Can you work these out from the model? Positions are in its coordinate system, mm. Give positions to 0.01 mm unless a question says otherwise; leave off trailing zeros. Order: outer loops, then holes, each group sorted by start corner. A loop starts at its lowest first (then second) coordinate and runs counter-clockwise, first axis right, second up. Notation, with made-up numbers: (-8.75, -37.75) - (22.25, -37.75) arc R27 cw to (22.25, -15.75) - close; hole circle Ø3 at (57, 33.25). An arc over 180 degrees is marked (long way). Answer as a JSON object with one key per item and string values.
```python
from build123d import *


with BuildPart() as f1:
    # F0 (on Top) → F1 (revolve)
    with BuildSketch(Plane.XY):
        with BuildLine():
            Line((-2.874578, 26.07), (0, 26.07))
            Line((0, 26.07), (0, 32))
            Line((0, 32), (0, 38.59))
            ThreePointArc((0, 38.59), (-6.422881, 33.474686), (-2.874578, 26.07))
        make_face()
        with BuildLine():
            Line((-8, 0), (0, 0))
            Line((0, 0), (0, 26.07))
            Line((0, 26.07), (-2.874578, 26.07))
            ThreePointArc((-2.874578, 26.07), (-3.059702, 17.543878), (-6.78, 9.87))
            Line((-6.78, 9.87), (-6.78, 6.87))
            Line((-6.78, 6.87), (-3.998394, 5.14))
            Line((-3.998394, 5.14), (-8, 2))
            Line((-8, 2), (-8, 0))
        make_face()
    revolve(axis=Axis((0, 19.295, 0), (0, 1, 0)))


solid = f1.part
```
Q1. If we section it at B-B, the plane y = 7.5: Please give me the cut outline in (x, z), then the cut area to 3 significant figures.
Recorded:
{"outline": "circle Ø13.56 at (0, 0)", "area": "144 mm^2"}
Q2. I need wall thicknesses on L1, parallel to Y at x = 3.5, z = 4.75; L2, parallel to Y at x = 1.25, z = -4.25 (3 decimals); L3, parallel to Z at x = 3.75, y = 30. Which ranges of each line are inside material? Lowest first, please.
Recorded:
{"L1": "y = 0 to 3.65, 6.32 to 11.08, 29.06 to 34.94", "L2": "y = 0 to 4.801, 5.408 to 13.665, 27.121 to 36.879", "L3": "z = -5.04 to 5.04"}
Q3. I'm going to push flat-ended pins straight in: pin 1 Ø1 at (x, y) = (5, 8.5) entering from +Z; pin 2 Ø8 at (x, z) = (-5, -3) entering from +Y; pin 3 Ø1 at (y, z) = (7.5, -0.5) entering from +X. Where does each tip first touch, or does it pass through?
Recorded:
{"pin 1": "stops at z = 5.07", "pin 2": "stops at y = 38.33", "pin 3": "stops at x = 6.78"}
Q4. If we section it at A-A, the plane z = 0: Please give me the cut outline in (x, y), then the cut area to 3 significant figures.
Recorded:
{"outline": "(-8, 0) - (8, 0) - (8, 2) - (4, 5.14) - (6.78, 6.87) - (6.78, 9.87) arc R20 cw to (2.87, 26.07) arc R6.59 ccw (long way) to (-2.87, 26.07) arc R20 cw to (-6.78, 9.87) - (-6.78, 6.87) - (-4, 5.14) - (-8, 2) - close", "area": "379 mm^2"}
Q5. We'd pull the mould along Y, two halves only. Please class faces 1 (the face through (1.73, 0.99, -7.81)), 2 (the face through (0.92, 4.94, -4.15)), 3 (the face through (0, 0, 0)): released by +Y, released by -Y, zero draft, split by the parting line, or undercut.
Recorded:
{"face 1": "zero draft", "face 2": "undercut", "face 3": "released by -Y"}
Q6. If we section it at D-D, the plane x = 5.25: Count the separate pieces of the cut face and the enclosed holes in it, then the cut area to 3 significant figures.
Recorded:
{"separate pieces": "3", "enclosed holes": "0", "area": "134 mm^2"}
Q7. If we section it at C-C, the plane x = 0: Please give me the cut outline in (y, z).
Recorded:
{"outline": "(0, -8) - (2, -8) - (5.14, -4) - (6.87, -6.78) - (9.87, -6.78) arc R20 cw to (26.07, -2.87) arc R6.59 ccw (long way) to (26.07, 2.87) arc R20 cw to (9.87, 6.78) - (6.87, 6.78) - (5.14, 4) - (2, 8) - (0, 8) - close"}
